Build history of the part. All positions in model axes, mm. Face numbers are marked on the shaded views. A direction names the side the tool comes from. Round coordinates to 2 decimals unless told otherwise and drop trailing zeros. Write each loop counter-clockwise with the first axis right and the second up, starting at its lowest first coordinate (ties: lowest second). Pieces come first, ordered by that corner, then holes. Notation, with made-up numbers: M -13,69 L -5,69 A32 cw -5,107 Z; hole C -13,2 d7. An arc over 180 degrees is marked long. Write item = value, one per line.
from build123d import *

# Parameters (mm, degrees)
SKETCH_1_W               = 60
SKETCH_1_H               = 40
EXTRUDE_1_DEPTH          = 100
SKETCH_6_R               = 20
EXTRUDE_2_DEPTH          = 20
EXTRUDE_START            = -20
SKETCH_7_R               = 20
EXTRUDE_3_DEPTH          = 20
CUT_EXTRUDE_1_DEPTH      = 120.268604419
CUT_EXTRUDE_1_DEPTH_BACK = 120.268604419
SKETCH_8_R               = 10
SKETCH_9_R               = 20
CUT_EXTRUDE_2_DEPTH      = 20
SKETCH_10_R              = 15
CUT_EXTRUDE_3_DEPTH      = 30
FILLET_2_R               = 2.5


with BuildPart() as part:
    # 스케치1 → 보스-돌출1 (new body)
    with BuildSketch(Plane.XY):
        with Locations((20, 5)):
            Rectangle(SKETCH_1_W, SKETCH_1_H)
    extrude(amount=EXTRUDE_1_DEPTH)

    # 스케치6 → 보스-돌출2 (add)
    with BuildSketch(Plane(origin=(50, 0, 0), x_dir=(0, 0, -1), z_dir=(1, 0, 0))):
        with Locations((0, 5)):
            Circle(SKETCH_6_R)
    extrude(amount=-EXTRUDE_2_DEPTH)

    # 스케치7 → 보스-돌출3 (add)
    with BuildSketch(Plane.ZY.offset(10).offset(EXTRUDE_START)):
        with Locations((0, 5)):
            Circle(SKETCH_7_R)
    extrude(amount=EXTRUDE_3_DEPTH)

    # 스케치8 → 컷-돌출1 (cut, two sides: drawn at the far end of the back side and taken through both)
    with BuildSketch(Plane.ZY.offset(10).offset(-CUT_EXTRUDE_1_DEPTH_BACK)):
        with Locations((0, 5)):
            Circle(SKETCH_8_R)
    extrude(amount=CUT_EXTRUDE_1_DEPTH + CUT_EXTRUDE_1_DEPTH_BACK, mode=Mode.SUBTRACT)

    # 스케치9 → 컷-돌출2 (cut)
    with BuildSketch(Plane.ZY.offset(-30)):
        with Locations((0, 5)):
            Circle(SKETCH_9_R)
    extrude(amount=CUT_EXTRUDE_2_DEPTH, mode=Mode.SUBTRACT)

    # 스케치10 → 컷-돌출3 (cut)
    with BuildSketch(Plane.XY.offset(100)):
        with Locations((20, 5)):
            Circle(SKETCH_10_R)
    extrude(amount=-CUT_EXTRUDE_3_DEPTH, mode=Mode.SUBTRACT)

    # 필렛2
    fillet_2_edges = [part.edges().sort_by_distance(p)[0] for p in [
        (5, 5, 100),
    ]]
    fillet(fillet_2_edges, radius=FILLET_2_R)


solid = part.part
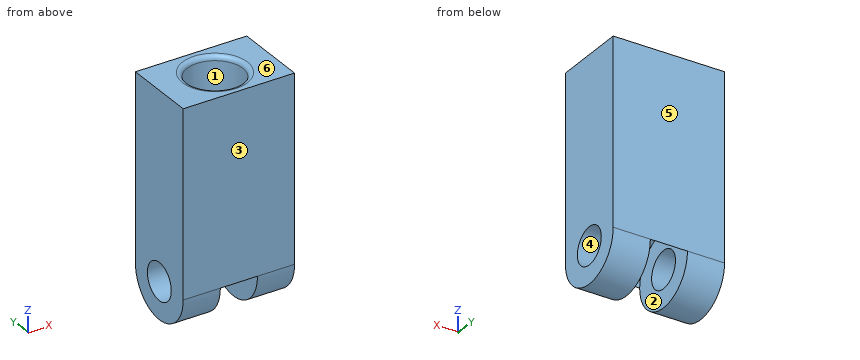
1. Band-saw the part on B-B (z = 78.5). List the corners of the cut face in (x, y).
Responses:
outline = M -10,-15 L 50,-15 L 50,25 L -10,25 Z; hole C 20,5 d30
2. Band-saw the part on C-C (x = 20). List the corners of the cut face in (y, z).
Responses:
outline = M -15,0 A20 cw 25,0 L 25,100 L 22.5,100 A2.5 ccw 20,97.5 L 20,70 L -10,70 L -10,97.5 A2.5 ccw -12.5,100 L -15,100 Z
3. Tool access for the marked faces 1, 2 and 3: list every direction of +Z, -Z, +X, -X, +Y, -Y with a clear straight run to the whole face (end or side of a thin tool).
Responses:
face_1 = +Z
face_2 = -Z
face_3 = +Z, -Z, +X, -X, -Y
4. Mould opens along Z. For the marked faces 4, 5 and 6 say: pulls with the +Z half, pulls with the -Z half, needs draft (parallel to the pull), parting line crosses it, or undercut.
Responses:
face_4 = undercut
face_5 = needs draft
face_6 = pulls with the +Z half
5. Band-saw the part on A-A (y = 5). List the corners of the cut face in (x, z).
Responses:
outline = M -10,-20 L 10,-20 L 10,-10 L -10,-10 Z; M -10,10 L 10,10 L 10,20 L 30,20 L 30,10 L 50,10 L 50,100 L 37.5,100 A2.5 ccw 35,97.5 L 35,70 L 5,70 L 5,97.5 A2.5 ccw 2.5,100 L -10,100 Z; M 30,-20 L 50,-20 L 50,-10 L 30,-10 Z
6. Band-saw the part on D-D (z = -8). List the corners of the cut face in (x, y).
Responses:
outline = M -10,-13.33 L 10,-13.33 L 10,-1 L -10,-1 Z; M -10,11 L 10,11 L 10,23.33 L -10,23.33 Z; M 30,-13.33 L 50,-13.33 L 50,-1 L 30,-1 Z; M 30,11 L 50,11 L 50,23.33 L 30,23.33 Z
7. Probe probe 1 along Y at (x, z) = (-4.25, 0); probe 2 along X at (y, z) = (16, -7.5); probe 3 along Y at (x, z) = (20, 76.25). List the from-to ranges inside material, lowest first.
Responses:
probe_1 = -15 to -5, 15 to 25
probe_2 = -10 to 10, 30 to 50
probe_3 = -15 to -10, 20 to 25
8. Flat gauge pins, fed straight in: pin 1 (8 mm diameter, centred on x = 12, y = -6, fed in from -Z); pin 2 (12 mm diameter, centred on x = 16.5, y = -3, fed in from -Z); pin 3 (9 mm diameter, centred on x = 18, y = 7, fed in from +Z); pin 4 (16 mm diameter, centred on y = 5, z = 0, fed in from +X). Where does each tip first touch, or does it go through?
Responses:
pin_1 = -18.53
pin_2 = 14.28
pin_3 = 70
pin_4 = through
